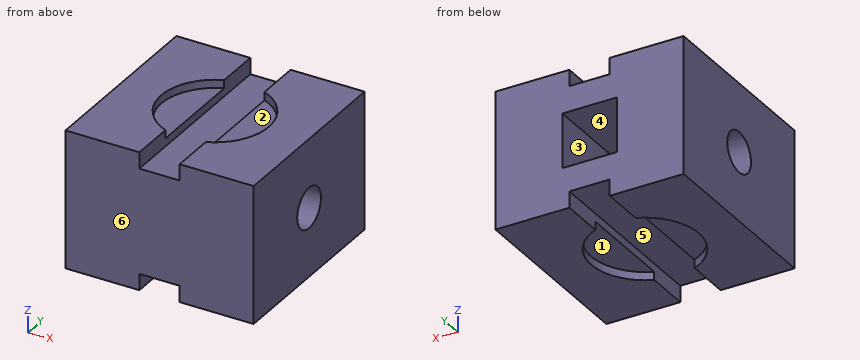
from build123d import *

# Parameters (mm, degrees)
SKETCH2_R           = 13.335
BOSS_EXTRUDE1_DEPTH = 2.032
SKETCH3_R           = 13.335
BOSS_EXTRUDE2_DEPTH = 2.032
BOSS_EXTRUDE3_START = -17.032
SKETCH5_W           = 46.67
SKETCH5_H           = 46.67
BOSS_EXTRUDE3_DEPTH = 34.064
SKETCH6_R           = 5
CUT_EXTRUDE1_DEPTH  = 55.888069277
SKETCH7_W           = 13.5
SKETCH7_H           = 13.5
CUT_EXTRUDE2_DEPTH  = 31.67
SKETCH9_W           = 10
SKETCH9_H           = 46.67
CUT_EXTRUDE3_DEPTH  = 4.032


with BuildPart() as part:
    # Sketch2 → Boss-Extrude1 (new body)
    with BuildSketch(Plane.XY.offset(15)):
        Circle(SKETCH2_R)
    extrude(amount=BOSS_EXTRUDE1_DEPTH)


with BuildPart() as body_2:
    # Sketch3 → Boss-Extrude2 (new body)
    with BuildSketch(Plane.XY.offset(-15)):
        Circle(SKETCH3_R)
    extrude(amount=-BOSS_EXTRUDE2_DEPTH)


with BuildPart() as body_3:
    # Sketch5 → Boss-Extrude3 (new body)
    with BuildSketch(Plane.XY.offset(BOSS_EXTRUDE3_START)):
        Rectangle(SKETCH5_W, SKETCH5_H)
    extrude(amount=BOSS_EXTRUDE3_DEPTH)

    # Sketch6 → Cut-Extrude1 (cut, through all)
    with BuildSketch(Plane.ZY.offset(23.335)):
        Circle(SKETCH6_R)
    extrude(amount=-CUT_EXTRUDE1_DEPTH, mode=Mode.SUBTRACT)

    # Sketch7 → Cut-Extrude2 (cut)
    with BuildSketch(Plane(origin=(0, 23.335, 0), x_dir=(1, 0, 0), z_dir=(0, 1, 0))):
        Rectangle(SKETCH7_W, SKETCH7_H)
    extrude(amount=-CUT_EXTRUDE2_DEPTH, mode=Mode.SUBTRACT)

    # Combine1: cut part, body 2
    add(part.part, mode=Mode.SUBTRACT)
    add(body_2.part, mode=Mode.SUBTRACT)

    # Sketch9 → Cut-Extrude3 (cut)
    with BuildSketch(Plane.XY.offset(17.032)):
        Rectangle(SKETCH9_W, SKETCH9_H)
    cut_extrude3 = extrude(amount=-CUT_EXTRUDE3_DEPTH, mode=Mode.SUBTRACT)

    # Mirror1: Cut-Extrude3 across plane
    add(cut_extrude3.mirror(Plane.XY), mode=Mode.SUBTRACT)


solid = body_3.part
Here's how the part is built. I have some questions about the finished solid (model axes, mm). Face numbers are marked on the shaded views. A direction names the side the tool comes from. Give positions to 0.01 mm unless a question says otherwise; leave off trailing zeros. Order: outer loops, then holes, each group sorted by start corner. A loop starts at its lowest first (then second) coordinate and runs counter-clockwise, first axis right, second up. Notation, with made-up numbers: M -19.75,40.5 L 34.25,40.5 A14 ccw 34.25,60.5 Z; hole C 49.25,28 d11. An arc over 180 degrees is marked long. Answer as a JSON object with one key per item and string values. Group by question number.
1) We'd pull the mould along Z, two halves only. Please class the marked faces 4, 5 and 6: pulls with the +Z half, pulls with the -Z half, needs draft (parallel to the pull), parting line crosses it, or undercut.
2) I'm going to push flat-ended pins straight in: pin 1 Ø4 at (x, y) = (8.5, 4) entering from +Z; pin 2 Ø2.5 at (x, y) = (10.5, -1) entering from -Z. Where does each tip first touch, or does it pass through?
3) Suppose I cut it at C-C, the plane y = 14.5. Write out the boundary of the cut face in (x, z) (3 decimals), plus the area to 3 significant figures.
4) Please list where these lines run through material, in increasing order: L1, parallel to Y at x = 18, z = 0 (3 decimals); L2, parallel to Z at x = -5.5, y = -5.5; L3, parallel to X at y = 5.5, z = 6 (3 decimals). Write a range as [from, to].
5) On a 3-axis mill with a long thin cutter (end or side, diameter ignored), from which of +Z, -Z, +X, -X, +Y, -Y can I reach the whole of each face in a straight line? I mean the marked faces 1, 2 and 3. Say none if no direction works.
6) Suppose I cut it at D-D, the plane z = 0. Write out the boundary of the cut face in (x, y) (3 decimals).
7) Suppose I cut it at A-A, the plane z = 4. Write out the boundary of the cut face in (x, y) (3 decimals), plus the area to 3 significant figures.
Results found:
{
 "1": {"face 4": "undercut", "face 5": "pulls with the -Z half", "face 6": "needs draft"},
 "2": {"pin 1": "z = 15", "pin 2": "z = -15"},
 "3": {"outline": "M -23.335,-17.032 L -5,-17.032 L -5,-13 L 5,-13 L 5,-17.032 L 23.335,-17.032 L 23.335,17.032 L 5,17.032 L 5,13 L -5,13 L -5,17.032 L -23.335,17.032 Z; hole M -6.75,-6.75 L 6.75,-6.75 L 6.75,6.75 L -6.75,6.75 Z", "area": "1,330 mm²"},
 "4": {"L1": "[-23.335, -5], [5, 23.335]", "L2": "[-15, -6.75], [6.75, 15]", "L3": "[-23.335, -6.75], [6.75, 23.335]"},
 "5": {"face 1": "-Z", "face 2": "+Z", "face 3": "+Y"},
 "6": {"outline": "M -23.335,-23.335 L 23.335,-23.335 L 23.335,-5 L 6.75,-5 L 6.75,-8.335 L -6.75,-8.335 L -6.75,-5 L -23.335,-5 Z; M -23.335,5 L -6.75,5 L -6.75,23.335 L -23.335,23.335 Z; M 6.75,5 L 23.335,5 L 23.335,23.335 L 6.75,23.335 Z"},
 "7": {"outline": "M -23.335,-23.335 L 23.335,-23.335 L 23.335,-3 L 6.75,-3 L 6.75,-8.335 L -6.75,-8.335 L -6.75,-3 L -23.335,-3 Z; M -23.335,3 L -6.75,3 L -6.75,23.335 L -23.335,23.335 Z; M 6.75,3 L 23.335,3 L 23.335,23.335 L 6.75,23.335 Z", "area": "1,550 mm²"}
}
